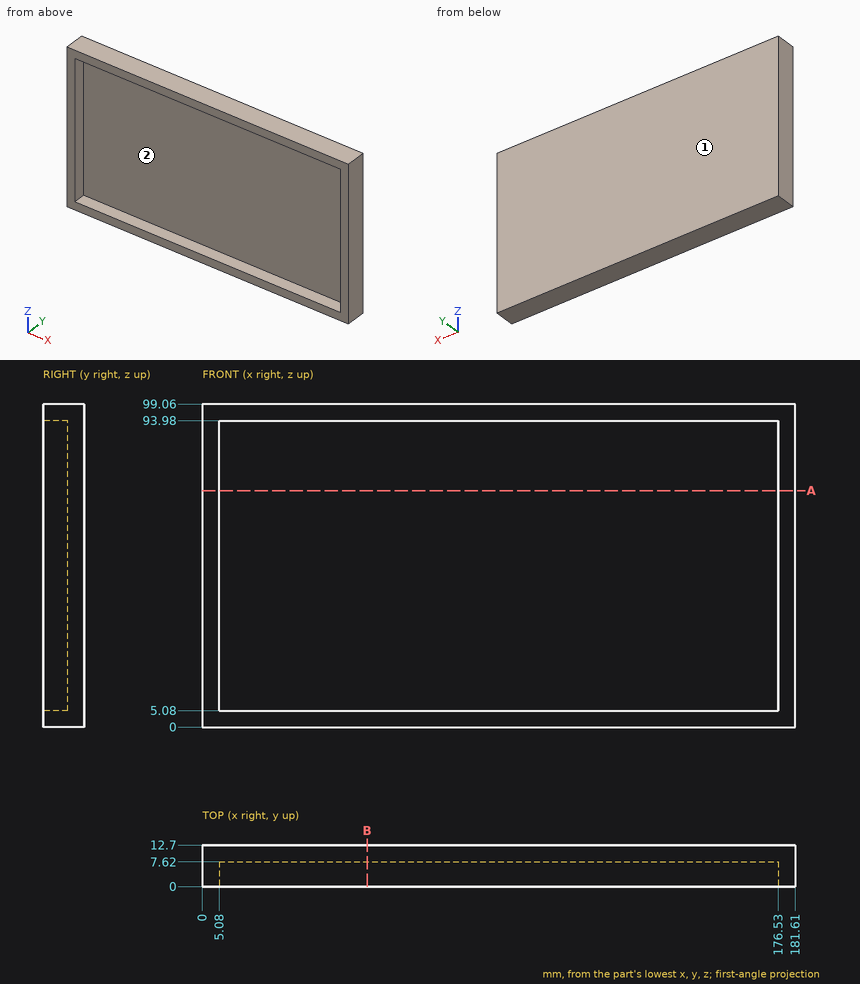
Check sheet for the drawn part. Datum: minimum x, y, z corner. Units: mm. Coordinates: 2 decimals unless noted, no trailing zeros. Loops run counter-clockwise (first coordinate to the right, second up) from the corner with the lowest first, then second, coordinate; pieces in that order, holes last. Notation, with made-up numbers: (83, 31) -> (96, 31) arc R28 ccw to (96, 60) -> close; hole circle Ø1 at (85, -30). An arc over 180 degrees is marked (long way). Answer as a JSON object with one key per item and string values. Group by question number.
Item 1: Mould release check, pull along Z, two halves, no side actions. Record for the marked faces 1 and 2: +Z half, -Z half, draft (parallel to the pull), parting line (faces both ways), or undercut.
Item 2: Sectioned sample at A-A on z = 72.5. Record the boundary of the cut face in (x, y), plus the area to 4 significant figures.
Item 3: Scan lines: probe 1 along Z at (x, y) = (82, 6.5); probe 2 along X at (y, z) = (3.5, 56); probe 3 along Y at (x, z) = (39, 54). Record each from-to range of solid material in increasing order.
Item 4: Depth check by flat-ended pin: pin 1 (5 mm diameter, centred on x = 81, z = 77.5, fed in from -Y). Enter the tip coordinate at first touch or a pass-through.
Item 5: Sectioned sample at B-B on x = 50.5. Record the boundary of the cut face in (y, z), plus the area to 3 significant figures.
Evaluation:
{
 "1": {"face 1": "draft", "face 2": "undercut"},
 "2": {"outline": "(0, 0) -> (5.08, 0) -> (5.08, 7.62) -> (176.53, 7.62) -> (176.53, 0) -> (181.61, 0) -> (181.61, 12.7) -> (0, 12.7) -> close", "area": "1,000 mm²"},
 "3": {"probe 1": "z = 0 to 5.08, 93.98 to 99.06", "probe 2": "x = 0 to 5.08, 176.53 to 181.61", "probe 3": "y = 7.62 to 12.7"},
 "4": {"pin 1": "stops at y = 7.62"},
 "5": {"outline": "(0, 0) -> (12.7, 0) -> (12.7, 99.06) -> (0, 99.06) -> (0, 93.98) -> (7.62, 93.98) -> (7.62, 5.08) -> (0, 5.08) -> close", "area": "581 mm²"}
}
